```python
from build123d import *

# Parameters (mm, degrees)
F0_R      = 1.5
F1_DEPTH  = 4
F2_W      = 14
F2_H      = 20
F3_DEPTH  = 26
F4_SIZE2  = 25.99999
F4_SIZE   = 1.49999
F5_W      = 10
F5_H      = 10
F6_DEPTH  = 5
F7_R      = 2.25
F8_DEPTH  = 25
F9_DEPTH  = 18
F10_W     = 10.5
F10_H     = 12
F11_DEPTH = 1
F13_W     = 8.5
F13_H     = 10
F13_W_2   = 1.9773303065
F13_H_2   = 4.2267278768
F14_DEPTH = 5
F15_SIZE  = 2.5


# Not quite as in the source:
# - a fillet or chamfer is up to 0.001 mm smaller than in the source, because OpenCascade refuses the exact size
# - a feature names something its author has since deleted; it is built from what else it names


with BuildPart() as f1:
    # F0 (on Top) → F1 (new body)
    with BuildSketch(Plane.XY):
        with BuildLine():
            Line((-8.25, 9), (8.25, 9))
            ThreePointArc((8.25, 9), (0, 17.25), (-8.25, 9))
        make_face()
        with Locations((0, 13.5)):
            Circle(F0_R, mode=Mode.SUBTRACT)
    extrude(amount=-F1_DEPTH)



with BuildPart() as f1b:
    # F0 (on Top) → F1, piece 2 (new body)
    with BuildSketch(Plane.XY):
        with BuildLine():
            ThreePointArc((-8.25, -9), (0, -17.25), (8.25, -9))
            Line((8.25, -9), (-8.25, -9))
        make_face()
        with Locations((0, -13.5)):
            Circle(F0_R, mode=Mode.SUBTRACT)
    extrude(amount=-F1_DEPTH)


with BuildPart() as f1_1:
    add(f1.part)

    add(f1b.part)  # F3 merges F1b
    # F2 (on face) → F3 (join)
    with BuildSketch(Plane(origin=(0, 0, -4), x_dir=(1, 0, 0), z_dir=(0, 0, -1))):
        Rectangle(F2_W, F2_H)
    extrude(amount=F3_DEPTH)

    # F4 (size 1.5 and 26 in the source; OpenCascade refuses exactly that, so slightly less here)
    f4_edges = [f1_1.edges().sort_by_distance(p)[0] for p in [
        (0, -10, -30),
        (0, 10, -30),
        (7, 0, -30),
        (-7, 0, -30),
    ]]
    f4_side = f1_1.faces().sort_by_distance((0, 0, -30))[0]
    chamfer(f4_edges, length=F4_SIZE, length2=F4_SIZE2, reference=f4_side)

    # F5 (on face) → F6 (join)
    with BuildSketch(Plane(origin=(0, 0, -30), x_dir=(1, 0, 0), z_dir=(0, 0, -1))):
        Rectangle(F5_W, F5_H)
    extrude(amount=F6_DEPTH)

    # F7 (on face) → F8 (join)
    with BuildSketch(Plane(origin=(0, 0, -35), x_dir=(1, 0, 0), z_dir=(0, 0, -1))):
        Circle(F7_R)
    extrude(amount=F8_DEPTH)

    # F9 (add): a face of the model
    f9_faces = [f1_1.faces().sort_by_distance(p)[0] for p in [
        (0, -9, -2),
    ]]
    extrude(f9_faces, amount=F9_DEPTH)

    # F10 (on face) → F11 (join)
    with BuildSketch(Plane.XY):
        Rectangle(F10_W, F10_H)
    extrude(amount=F11_DEPTH)

    # F13 (on face) → F14 (cut)
    with BuildSketch(Plane.XY.offset(1)):
        Rectangle(F13_W, F13_H)
        Rectangle(F13_W_2, F13_H_2, mode=Mode.SUBTRACT)
    extrude(amount=-F14_DEPTH, mode=Mode.SUBTRACT)

    # F15
    f15_edges = [f1_1.edges().sort_by_distance(p)[0] for p in [
        (-4.25, -5, -1.5),
        (-4.25, 5, -1.5),
    ]]
    chamfer(f15_edges, length=F15_SIZE)


solid = f1_1.part
```
The listing builds one solid part. Answer for the finished solid, in the listing's coordinates (mm). A direction names the side the tool comes from. Give positions to 0.01 mm unless a question says otherwise; leave off trailing zeros. Order: outer loops, then holes, each group sorted by start corner. A loop starts at its lowest first (then second) coordinate and runs counter-clockwise, first axis right, second up. Notation, with made-up numbers: (53.5, 72.5) -> (63.5, 72.5) arc R19 cw to (63.5, 93.5) -> close; hole circle Ø7 at (66.5, -37.5). An arc over 180 degrees is marked (long way). One line per item, written item: value.
1) A tool of negligible diameter and unlimited length cuts with its end or side. For faces 1 (the flat face through (-1.2, -2.3, -35)), 2 (the flat face through (0, -5, -32)), 3 (the flat face through (4.25, 0, -1)), from which of +Z, -Z, +X, -X, +Y, -Y can it reach the whole face along a straight path? Write none if from no direction.
Reported:
face 1: -Z
face 2: -Z, +X, -X, -Y
face 3: +Z
2) Flat-ended cylindrical pins translate along their axes: P1, Ø3, axis at y = -6, z = -8, coming from the +X side; P2, Ø2.5, axis at y = 2, z = -31.5, coming from the -X side; P3, Ø5.5, axis at x = -0.5, z = -32.5, coming from the +Y side; P4, Ø3, axis at x = -5.5, z = -38.5, coming from the +Y side. Find the tip coordinate at first contact, or state that the pin passes through.
Reported:
P1: stops at x = 6.86
P2: stops at x = -5
P3: stops at y = 8.51
P4: passes through
3) Find section B-B, the plane x = 0. Count the separate pieces of the cut face and the enclosed holes in it, plus the area to 3 significant figures.
Reported:
separate pieces: 3
enclosed holes: 0
area: 741 mm^2
4) Determine the mould class of faces 4 (the flat face through (1, -5, -1)), 5 (the flat face through (8.25, 0, -2)), 6 (the cylindrical face through (0.18, 17.25, -1.97)) for opening direction Y: pulls with the +Y half, pulls with the -Y half, needs draft (parallel to the pull), parting line crosses it, or undercut.
Reported:
face 4: undercut
face 5: needs draft
face 6: pulls with the +Y half
5) Find section C-C, the plane y = 13.5. Determine the outline of the cut face in (x, z), plus the area to 3 significant figures.
Reported:
outline: (-6.91, -4) -> (-1.5, -4) -> (-1.5, 0) -> (-6.91, 0) -> close; (1.5, -4) -> (6.91, -4) -> (6.91, 0) -> (1.5, 0) -> close
area: 43.3 mm^2
6) Find the intervals of material crossed by line 1 (Y direction, x = 0, z = -1.8); line 2 (Z direction, x = -2.5, y = -11.5); line 3 (X direction, y = 4.5, z = -31), in increasing order.
Reported:
line 1: y = -17.25 to -15, -12 to -5, -2.11 to 2.11, 5 to 12, 15 to 17.25
line 2: z = -4 to 0
line 3: x = -5 to 5
